Read the model definition and answer for the solid it produces. Units are mm, in the model's axes. Face numbers are marked on the shaded views. A direction names the side the tool comes from. Coordinates: 2 decimals unless noted, no trailing zeros. Write each loop counter-clockwise with the first axis right and the second up, starting at its lowest first coordinate (ties: lowest second). Pieces come first, ordered by that corner, then holes.
1) Each of these flat-tipped pins is pushed along its axis until it touches: pin 1 Ø4 at (x, y) = (-3, -9) entering from -Z; pin 2 Ø2 at (y, z) = (7.5, 9) entering from +X. Where does it stop, or does it pass through?
2) Which of the six approach directions +Z, -Z, +X, -X, +Y, -Y give full straight-line access (tool end or side, diameter ignored) to the marked faces 4 and 5?
3) The part is cut by section D-D (z = 15). Determine the outline of the cut face in (x, y), then the cut area to 3 significant figures.
4) The part is cut by section C-C (x = -4). Determine the outline of the cut face in (y, z).
5) The part is cut by section B-B (y = 2.35). Determine the outline of the cut face in (x, z), then the cut area to 3 significant figures.
6) Find the intervals of material crossed by line 1 (Y direction, x = 0, z = 2.5); line 2 (Y direction, x = -1.25, z = 10); line 3 (Y direction, x = -2, z = 3.5), in increasing order.
7) The part is cut by section A-A (z = 9.5). Determine the outline of the cut face in (x, y), then the cut area to 3 significant figures.
8) Determine the mould class of the marked faces 1, 2 and 3 for opening direction X: +X half, -X half, draft (parallel to the pull), parting line (faces both ways), or undercut.
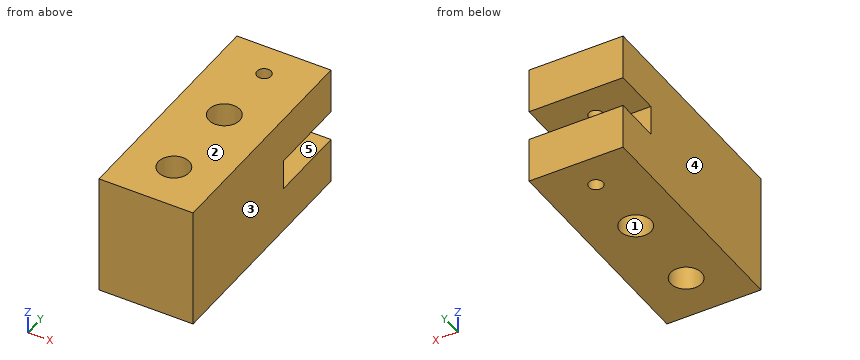
from build123d import *

# Parameters (mm, degrees)
SKETCH2_W           = 14
SKETCH2_H           = 34.7
BOSS_EXTRUDE1_DEPTH = 18
SKETCH3_R           = 2.3
CUT_EXTRUDE1_DEPTH  = 26.961943302
SKETCH4_W           = 4.5
SKETCH4_H           = 12
CUT_EXTRUDE2_DEPTH  = 8
SKETCH5_R           = 1.05
CUT_EXTRUDE3_DEPTH  = 26.961943302
SKETCH8_W           = 4.5
SKETCH8_H           = 7
CUT_EXTRUDE6_DEPTH  = 29.653490189


with BuildPart() as part:
    # Sketch2 → Boss-Extrude1 (new body)
    with BuildSketch(Plane.XY):
        Rectangle(SKETCH2_W, SKETCH2_H)
    extrude(amount=BOSS_EXTRUDE1_DEPTH)

    # Sketch3 → Cut-Extrude1 (cut, through all)
    with BuildSketch(Plane.XY.offset(18)):
        with Locations((0, -10.35)):
            Circle(SKETCH3_R)
        with Locations((0, 2.35)):
            Circle(SKETCH3_R)
    extrude(amount=-CUT_EXTRUDE1_DEPTH, mode=Mode.SUBTRACT)

    # Sketch4 → Cut-Extrude2 (cut)
    with BuildSketch(Plane(origin=(7, 0, 0), x_dir=(0, 0, -1), z_dir=(1, 0, 0))):
        with Locations((-9, 11.35)):
            Rectangle(SKETCH4_W, SKETCH4_H)
    extrude(amount=-CUT_EXTRUDE2_DEPTH, mode=Mode.SUBTRACT)

    # Sketch5 → Cut-Extrude3 (cut, through all)
    with BuildSketch(Plane.XY.offset(18)):
        with Locations((0, 12.35)):
            Circle(SKETCH5_R)
    extrude(amount=-CUT_EXTRUDE3_DEPTH, mode=Mode.SUBTRACT)

    # Sketch8 → Cut-Extrude6 (cut, through all)
    with BuildSketch(Plane(origin=(7, 0, 0), x_dir=(0, 0, -1), z_dir=(1, 0, 0))):
        with Locations((-9, 13.85)):
            Rectangle(SKETCH8_W, SKETCH8_H)
    extrude(amount=-CUT_EXTRUDE6_DEPTH, mode=Mode.SUBTRACT)


solid = part.part
Reported:
1. pin 1: stops at z = 0
1. pin 2: stops at x = -1
2. face 4: +Z, -Z, -X, +Y, -Y
2. face 5: +X, +Y
3. outline: (-7, -17.35) - (7, -17.35) - (7, 17.35) - (-7, 17.35) - close; hole circle Ø4.6 at (0, -10.35); hole circle Ø4.6 at (0, 2.35); hole circle Ø2.1 at (0, 12.35)
3. area: 449 mm2
4. outline: (-17.35, 0) - (17.35, 0) - (17.35, 6.75) - (10.35, 6.75) - (10.35, 11.25) - (17.35, 11.25) - (17.35, 18) - (-17.35, 18) - close
5. outline: (-7, 0) - (-2.3, 0) - (-2.3, 18) - (-7, 18) - close; (2.3, 0) - (7, 0) - (7, 18) - (2.3, 18) - close
5. area: 169 mm2
6. line 1: y = -17.35 to -12.65, -8.05 to 0.05, 4.65 to 11.3, 13.4 to 17.35
6. line 2: y = -17.35 to -12.28, -8.42 to 0.42, 4.28 to 10.35
6. line 3: y = -17.35 to -11.49, -9.21 to 1.21, 3.49 to 17.35
7. outline: (-7, -17.35) - (7, -17.35) - (7, 5.35) - (-1, 5.35) - (-1, 10.35) - (-7, 10.35) - close; hole circle Ø4.6 at (0, -10.35); hole circle Ø4.6 at (0, 2.35)
7. area: 315 mm2
8. face 1: undercut
8. face 2: draft
8. face 3: +X half
